CAD build for the part. Positions are in the model's coordinates, mm. Face numbers are marked on the shaded views. A direction names the side the tool comes from. Give positions to 0.01 mm unless a question says otherwise; leave off trailing zeros. Loops run counter-clockwise (first coordinate to the right, second up) from the corner with the lowest first, then second, coordinate; pieces in that order, holes last. Notation, with made-up numbers: (50.25, 5.5) -> (88.25, 5.5) arc R5 ccw to (88.25, 11.5) -> close; hole circle Ø9 at (30, 16). An arc over 180 degrees is marked (long way). Use one line per item in the form item = value.
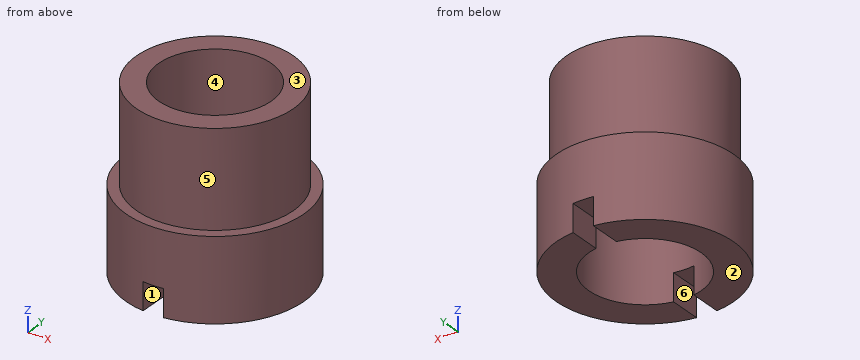
```python
from build123d import *

# Parameters (mm, degrees)
SKETCH1_R               = 10.3124
SKETCH1_R_2             = 6.5405
BOSS_EXTRUDE1_DEPTH     = 4.7625
SKETCH2_R               = 9.1186
SKETCH2_R_2             = 6.5405
BOSS_EXTRUDE2_DEPTH     = 11.0998
SKETCH3_W               = 2.3622
SKETCH3_H               = 3.175
CUT_EXTRUDE1_DEPTH      = 11.3124
CUT_EXTRUDE1_DEPTH_BACK = 11.3124


with BuildPart() as part:
    # Sketch1 → Boss-Extrude1 (new body, symmetric)
    with BuildSketch(Plane.XY):
        Circle(SKETCH1_R)
        Circle(SKETCH1_R_2, mode=Mode.SUBTRACT)
    extrude(amount=BOSS_EXTRUDE1_DEPTH, both=True)

    # Sketch2 → Boss-Extrude2 (add)
    with BuildSketch(Plane.XY.offset(4.7625)):
        Circle(SKETCH2_R)
        Circle(SKETCH2_R_2, mode=Mode.SUBTRACT)
    extrude(amount=BOSS_EXTRUDE2_DEPTH)

    # Sketch3 → Cut-Extrude1 (cut, two sides)
    with BuildSketch(Plane(origin=(0, 0, 0), x_dir=(1, 0, 0), z_dir=(0, 1, 0))) as cut_extrude1_sk:
        with Locations((0, 3.175)):
            Rectangle(SKETCH3_W, SKETCH3_H)
    extrude(amount=CUT_EXTRUDE1_DEPTH, mode=Mode.SUBTRACT)
    extrude(cut_extrude1_sk.sketch, amount=-CUT_EXTRUDE1_DEPTH_BACK, mode=Mode.SUBTRACT)


solid = part.part
```
1. Cut at C-C, the plane z = 12.75. Write the cut outline in (x, y), then the cut area to 3 significant figures.
Result sheet:
outline = circle Ø18.24 at (0, 0); hole circle Ø13.08 at (0, 0)
area = 127 mm^2
2. Cut at A-A, the plane y = 0. Write the cut outline in (x, z).
Result sheet:
outline = (-10.31, -4.76) -> (-6.54, -4.76) -> (-6.54, 15.86) -> (-9.12, 15.86) -> (-9.12, 4.76) -> (-10.31, 4.76) -> close; (6.54, -4.76) -> (10.31, -4.76) -> (10.31, 4.76) -> (9.12, 4.76) -> (9.12, 15.86) -> (6.54, 15.86) -> close
3. Cut at B-B, the plane x = 0. Write the cut outline in (y, z), then the cut area to 3 significant figures.
Result sheet:
outline = (-10.31, -1.59) -> (-6.54, -1.59) -> (-6.54, 15.86) -> (-9.12, 15.86) -> (-9.12, 4.76) -> (-10.31, 4.76) -> close; (6.54, -1.59) -> (10.31, -1.59) -> (10.31, 4.76) -> (9.12, 4.76) -> (9.12, 15.86) -> (6.54, 15.86) -> close
area = 105 mm^2
4. Drop flat-ended pins along their axis: P1, Ø4, axis at x = 1.5, z = 10.5, coming from the -Y side; P2, Ø2.5, axis at y = 8.5, z = -3, coming from the -X side; P3, Ø10, axis at y = 7.5, z = -1, coming from the +X side; P4, Ø1, axis at x = 0, y = -5, coming from the +Z side. Give the stop position or say it passes through.
Result sheet:
P1 = -9.12
P2 = -7.33
P3 = 10
P4 = through
5. Drill centre lines: line 1 (Y direction, x = 0, z = 9); line 2 (X direction, y = 0, z = 2.5); line 3 (Z direction, x = -6.75, y = -6.75). Where is each one in solid material? Low to high.
Result sheet:
line_1 = -9.12 to -6.54, 6.54 to 9.12
line_2 = -10.31 to -6.54, 6.54 to 10.31
line_3 = -4.76 to 4.76
6. Mould opens along X. For the marked faces 3, 4, 5 and 6 say: pulls with the +X half, pulls with the -X half, needs draft (parallel to the pull), parting line crosses it, or undercut.
Result sheet:
face_3 = needs draft
face_4 = undercut
face_5 = parting line crosses it
face_6 = undercut
7. Tool access for the marked faces 1 and 2: list every direction of +Z, -Z, +X, -X, +Y, -Y with a clear straight run to the whole face (end or side of a thin tool).
Result sheet:
face_1 = -Z, +Y, -Y
face_2 = -Z, +X, -X, +Y, -Y
